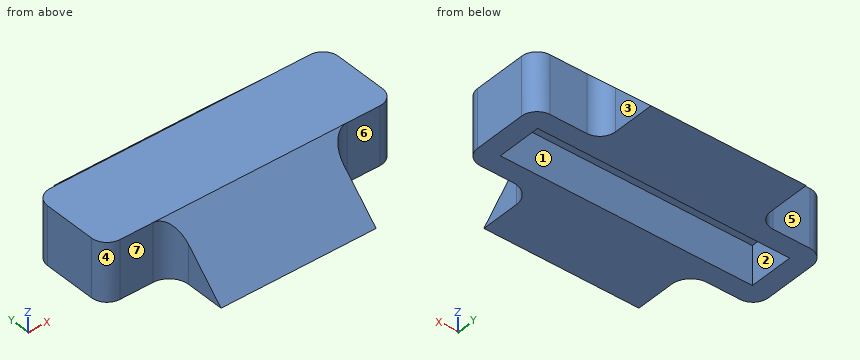
```python
from build123d import *

# Parameters (mm, degrees)
F0_W      = 190.5
F0_H      = 54.61
F1_DEPTH  = 38.1
F2_W      = 165.1
F2_H      = 29.21
F3_DEPTH  = 25.4
F4_W      = 101.6
F4_H      = 38.1
F5_DEPTH  = 38.1
F6_SIZE   = 38.09999
F7_R      = 10.16
F8_R      = 10.16
F9_W      = 101.6
F9_H      = 38.1
F10_DEPTH = 38.1
F11_SIZE  = 38.09999
F12_R     = 12.7


# Not quite as in the source:
# - a fillet or chamfer is up to 0.001 mm smaller than in the source, because OpenCascade refuses the exact size


with BuildPart() as f1:
    # F0 (on Top) → F1 (new body)
    with BuildSketch(Plane.XY):
        Rectangle(F0_W, F0_H)
    extrude(amount=F1_DEPTH)

    # F2 (on face) → F3 (cut)
    with BuildSketch(Plane(origin=(0, 0, 0), x_dir=(1, 0, 0), z_dir=(0, 0, -1))):
        Rectangle(F2_W, F2_H)
    extrude(amount=-F3_DEPTH, mode=Mode.SUBTRACT)

    # F4 (on face) → F5 (join)
    with BuildSketch(Plane(origin=(0, 27.305, 0), x_dir=(-1, 0, 0), z_dir=(0, 1, 0))):
        with Locations((0, 19.05)):
            Rectangle(F4_W, F4_H)
    extrude(amount=F5_DEPTH)

    # F6 (size 38.1 in the source; OpenCascade refuses exactly that, so slightly less here)
    f6_edges = [f1.edges().sort_by_distance(p)[0] for p in [
        (0, 65.405, 38.1),
    ]]
    chamfer(f6_edges, length=F6_SIZE)

    # F7 (call 1 of 2: OpenCascade refuses the feature's edges together)
    f7_edges = [f1.edges().sort_by_distance(p)[0] for p in [
        (-50.8, 27.305, 19.05),
    ]]
    fillet(f7_edges, radius=F7_R)

    # F7#2 (call 2 of 2)
    f7_2_edges = [f1.edges().sort_by_distance(p)[0] for p in [
        (50.8, 27.305, 19.05),
    ]]
    fillet(f7_2_edges, radius=F7_R)

    # F8
    f8_edges = [f1.edges().sort_by_distance(p)[0] for p in [
        (-95.25, 27.305, 19.05),
        (-95.25, -27.305, 19.05),
        (95.25, 27.305, 19.05),
        (95.25, -27.305, 19.05),
    ]]
    fillet(f8_edges, radius=F8_R)

    # F9 (on face) → F10 (join)
    with BuildSketch(Plane.XZ.offset(27.305)):
        with Locations((0, 19.05)):
            Rectangle(F9_W, F9_H)
    extrude(amount=F10_DEPTH)

    # F11 (size 38.1 in the source; OpenCascade refuses exactly that, so slightly less here)
    f11_edges = [f1.edges().sort_by_distance(p)[0] for p in [
        (0, -65.405, 38.1),
    ]]
    chamfer(f11_edges, length=F11_SIZE)

    # F12 (call 1 of 2: OpenCascade refuses the feature's edges together)
    f12_edges = [f1.edges().sort_by_distance(p)[0] for p in [
        (50.8, -27.305, 19.05),
    ]]
    fillet(f12_edges, radius=F12_R)

    # F12#2 (call 2 of 2)
    f12_2_edges = [f1.edges().sort_by_distance(p)[0] for p in [
        (-50.8, -27.305, 19.05),
    ]]
    fillet(f12_2_edges, radius=F12_R)


solid = f1.part
```
Geometry: final body of the model. Coordinates: model frame, mm. Face numbers are marked on the shaded views. A direction names the side the tool comes from. Coordinates: 2 decimals unless noted, no trailing zeros. Order: outer loops, then holes, each group sorted by start corner. A loop starts at its lowest first (then second) coordinate and runs counter-clockwise, first axis right, second up.
Item 1: Draft query along Y for the marked faces 1, 2, 3 and 4. Return one class per face: released by +Y, released by -Y, zero draft, split by the parting line, or undercut.
Answer:
face 1: undercut
face 2: undercut
face 3: zero draft
face 4: released by -Y
Item 2: Section query D-D (z = 31). Output: boundary loops of the cut face in (x, y) (3 decimals).
Answer:
outline: (-95.25, -17.145) arc R10.16 ccw to (-85.09, -27.305) - (-63.5, -27.305) arc R12.7 cw to (-52.101, -34.405) - (52.101, -34.405) arc R12.7 cw to (63.5, -27.305) - (85.09, -27.305) arc R10.16 ccw to (95.25, -17.145) - (95.25, 17.145) arc R10.16 ccw to (85.09, 27.305) - (60.96, 27.305) arc R10.16 cw to (51.272, 34.405) - (-51.272, 34.405) arc R10.16 cw to (-60.96, 27.305) - (-85.09, 27.305) arc R10.16 ccw to (-95.25, 17.145) - close
Item 3: Material intervals for line 1 along X through (y, z) = (0.5, 2); line 2 along Y through (x, z) = (-80, 20.5) (3 decimals); line 3 along Y through (x, z) = (79.5, 28) (3 decimals), sorted ascending.
Answer:
line 1: x = -95.25 to -82.55, 82.55 to 95.25
line 2: y = -27.305 to -14.605, 14.605 to 27.305
line 3: y = -27.305 to 27.305
Item 4: Section query A-A (y = 9.5). Output: boundary loops of the cut face in (x, z), then the cut area to 3 significant figures.
Answer:
outline: (-95.25, 0) - (-82.55, 0) - (-82.55, 25.4) - (82.55, 25.4) - (82.55, 0) - (95.25, 0) - (95.25, 38.1) - (-95.25, 38.1) - close
area: 3,060 mm2
Item 5: Contact query for flat-ended pins moving along their axis: P1, Ø12, axis at y = 28.5, z = 31, coming from the -X side; P2, Ø2, axis at x = 11.5, z = 22, coming from the -Y side (3 decimals); P3, Ø7, axis at x = -77, z = 24.5, coming from the +Y side (3 decimals). Output: stop coordinate, or through.
Answer:
P1: stops at x = -93.72
P2: stops at y = -44.405
P3: stops at y = 27.305
Item 6: Access query for the marked faces 5, 6 and 7. Directions: +Z, -Z, +X, -X, +Y, -Y. A direction counts if a zero-diameter tool reaches every point of the face in a straight line with its end or side. Return the directions, or none.
Answer:
face 5: +Z, -Z, -X, +Y
face 6: +Z, -Z, +X, -Y
face 7: +Z, -Z, -X, -Y
Item 7: Section query B-B (z = 3.5). Output: boundary loops of the cut face in (x, y) (3 decimals), then the cut area to 3 significant figures.
Answer:
outline: (-95.25, -17.145) arc R10.16 ccw to (-85.09, -27.305) - (-63.5, -27.305) arc R12.7 cw to (-50.8, -40.005) - (-50.8, -61.905) - (50.8, -61.905) - (50.8, -40.005) arc R12.7 cw to (63.5, -27.305) - (85.09, -27.305) arc R10.16 ccw to (95.25, -17.145) - (95.25, 17.145) arc R10.16 ccw to (85.09, 27.305) - (60.96, 27.305) arc R10.16 cw to (50.8, 37.465) - (50.8, 61.905) - (-50.8, 61.905) - (-50.8, 37.465) arc R10.16 cw to (-60.96, 27.305) - (-85.09, 27.305) arc R10.16 ccw to (-95.25, 17.145) - close; hole (-82.55, -14.605) - (82.55, -14.605) - (82.55, 14.605) - (-82.55, 14.605) - close
area: 12,600 mm2
